from build123d import *

# Parameters (mm, degrees)
BOX001_W     = 80
BOX001_H     = 80
BOX001_DEPTH = 64
FILLET_R     = 12
THICKNESS_T  = 3


with BuildPart() as part:
    # Box001 → Box001 (new body)
    with BuildSketch(Plane.XY):
        with Locations((40, 40)):
            Rectangle(BOX001_W, BOX001_H)
    extrude(amount=BOX001_DEPTH)

    # Fillet
    fillet_edges = [part.edges().sort_by_distance(p)[0] for p in [
        (0, 0, 32),
        (0, 80, 32),
        (80, 0, 32),
        (80, 80, 32),
    ]]
    fillet(fillet_edges, radius=FILLET_R)

    # Thickness
    thickness_openings = [part.faces().sort_by_distance(p)[0] for p in [
        (40, 40, 0),
    ]]
    offset(amount=THICKNESS_T, openings=thickness_openings)


solid = part.part
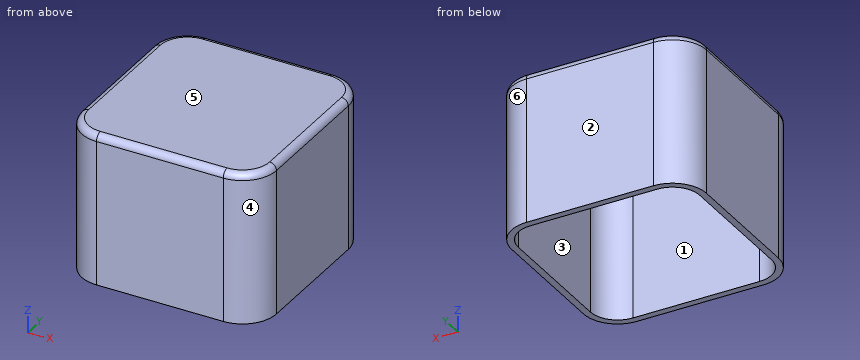
Input: part model. Units: mm. Frame: model coordinates. Face numbers are marked on the shaded views. A direction names the side the tool comes from. Coordinates: 2 decimals unless noted, no trailing zeros. Order: outer loops, then holes, each group sorted by start corner. A loop starts at its lowest first (then second) coordinate and runs counter-clockwise, first axis right, second up. Notation, with made-up numbers: M 48,50 L 78,50 A30 cw 78,75 Z; hole C -21,35 d10. An arc over 180 degrees is marked long. Write item = value, one per line. Start each with the question number.
(1) Reachability of the marked faces 1 and 2 from +Z, -Z, +X, -X, +Y, -Y: full face, straight path, thin tool, end or side. Return the list, or none.
(2) Section B-B on y = 23. Output: boundary loops of the cut face in (x, z), and give its area (3 significant figures).
(3) Section A-A on z = 47. Output: boundary loops of the cut face in (x, y).
(4) Pull-direction query (Y, two-part tool) for the marked faces 3, 4, 5 and 6; classes: released by +Y, released by -Y, zero draft, split by the parting line, or undercut.
(5) First-contact query: P1, Ø24, axis at x = 49.5, y = 46.5, coming from the -Z side. Flat tip, straight axial feed; report the tip coordinate or a pass-through.
(6) Line query: line 1 along X through (y, z) = (50, 27.5); line 2 along Z through (x, y) = (79.5, 18.5). Output: solid intervals per line, ascending. Write a range as [from, to].
Result set:
q1.face_1 = -Z
q1.face_2 = +Z, -Z, +X, -X, +Y
q2.outline = M -3,0 L 0,0 L 0,64 L 80,64 L 80,0 L 83,0 L 83,64 A3 ccw 80,67 L 0,67 A3 ccw -3,64 Z
q2.area = 638 mm²
q3.outline = M -3,12 A15 ccw 12,-3 L 68,-3 A15 ccw 83,12 L 83,68 A15 ccw 68,83 L 12,83 A15 ccw -3,68 Z; hole M 0,12 A12 ccw 12,0 L 68,0 A12 ccw 80,12 L 80,68 A12 ccw 68,80 L 12,80 A12 ccw 0,68 Z
q4.face_3 = undercut
q4.face_4 = released by -Y
q4.face_5 = zero draft
q4.face_6 = released by +Y
q5.P1 = 64
q6.line_1 = [-3, 0], [80, 83]
q6.line_2 = [64, 67]
